```python
from build123d import *

# Parameters (mm, degrees)
SALIENTE_EXTRUIR1_DEPTH = 40
VACIADO1_T              = -1
SALIENTE_EXTRUIR3_START = 2
SALIENTE_EXTRUIR3_DEPTH = 2
CROQUIS5_R              = 3.75
CORTAR_EXTRUIR2_DEPTH   = 2.5
SALIENTE_EXTRUIR5_DEPTH = 5
CORTAR_EXTRUIR3_DEPTH   = 6
CORTAR_EXTRUIR4_DEPTH   = 1
CORTAR_EXTRUIR5_DEPTH   = 1


with BuildPart() as part:
    # Croquis1 → Saliente-Extruir1 (new body)
    with BuildSketch(Plane(origin=(0, 0, 0), x_dir=(1, 0, 0), z_dir=(0, 1, 0))):
        with BuildLine():
            Line((-25, 0), (-69.8, 0))
            ThreePointArc((-69.8, 0), (-64.717433049, 26.14754022), (-50.209918064, 48.487154258))
            Line((-50.209918064, 48.487154258), (-17.983495008, 17.366459261))
            ThreePointArc((-17.983495008, 17.366459261), (-23.179596364, 9.365164835), (-25, 0))
        make_face()
    extrude(amount=SALIENTE_EXTRUIR1_DEPTH)

    # Vaciado1
    vaciado1_openings = [part.faces().sort_by_distance(p)[0] for p in [
        (-46.068338787, 40, -18.61281705),
    ]]
    offset(amount=VACIADO1_T, openings=vaciado1_openings, kind=Kind.INTERSECTION)

    # Croquis4 → Saliente-Extruir3 (add)
    with BuildSketch(Plane.XZ.offset(SALIENTE_EXTRUIR3_START)):
        with BuildLine():
            Line((-25, 0), (-69.8, 0))
            ThreePointArc((-69.8, 0), (-64.717433049, -26.14754022), (-50.209918064, -48.487154258))
            Line((-50.209918064, -48.487154258), (-17.983495008, -17.366459261))
            ThreePointArc((-17.983495008, -17.366459261), (-23.179596364, -9.365164835), (-25, 0))
        make_face()
    extrude(amount=-SALIENTE_EXTRUIR3_DEPTH)

    # Croquis5 → Cortar-Extruir2 (cut)
    with BuildSketch(Plane(origin=(0, 1, 0), x_dir=(1, 0, 0), z_dir=(0, 1, 0))):
        with Locations(Location((-55.631031274, 22.476395605, 0), (0, 0, 270))):
            Circle(CROQUIS5_R)
    extrude(amount=-CORTAR_EXTRUIR2_DEPTH, mode=Mode.SUBTRACT)

    # Croquis6 → Saliente-Extruir5 (add)
    with BuildSketch(Plane(origin=(0, 1, 0), x_dir=(1, 0, 0), z_dir=(0, 1, 0))):
        with BuildLine():
            Line((-25, 0), (-50, 0))
            ThreePointArc((-50, 0), (-46.359192728, 18.730329671), (-35.966990017, 34.732918523))
            Line((-35.966990017, 34.732918523), (-17.983495008, 17.366459261))
            ThreePointArc((-17.983495008, 17.366459261), (-23.179596364, 9.365164835), (-25, 0))
        make_face()
    extrude(amount=SALIENTE_EXTRUIR5_DEPTH)

    # Croquis2 → Cortar-Extruir3 (cut)
    with BuildSketch(Plane(origin=(0, -2, 0), x_dir=(1, 0, 0), z_dir=(0, 1, 0))):
        with BuildLine():
            Line((-39.728874148, 27.818457163), (-29.899049617, 20.935539927))
            ThreePointArc((-29.899049617, 20.935539927), (-33.842210692, 13.67314066), (-36.050624432, 5.709857974))
            Line((-36.050624432, 5.709857974), (-47.902884519, 7.587071554))
            ThreePointArc((-47.902884519, 7.587071554), (-44.968416946, 18.168419781), (-39.728874148, 27.818457163))
        make_face()
    extrude(amount=CORTAR_EXTRUIR3_DEPTH, mode=Mode.SUBTRACT)

    # Croquis7 → Cortar-Extruir4 (cut)
    with BuildSketch(Plane.XY):
        Polygon((-62.8, 38), (-67.8, 35.113248654), (-67.8, 29.339745962), (-62.8, 26.452994616), (-57.8, 29.339745962), (-57.8, 35.113248654), align=None)
        Polygon((-47.8, 38), (-52.8, 35.113248654), (-52.8, 29.339745962), (-47.8, 26.452994616), (-42.8, 29.339745962), (-42.8, 35.113248654), align=None)
        Polygon((-32.8, 38), (-37.8, 35.113248654), (-37.8, 29.339745962), (-32.8, 26.452994616), (-27.8, 29.339745962), (-27.8, 35.113248654), align=None)
        Polygon((-47.8, 12.983724512), (-52.8, 10.096973166), (-52.8, 4.323470474), (-47.8, 1.436719129), (-42.8, 4.323470474), (-42.8, 10.096973166), align=None)
        Polygon((-32.8, 12.983724512), (-37.8, 10.096973166), (-37.8, 4.323470474), (-32.8, 1.436719129), (-27.8, 4.323470474), (-27.8, 10.096973166), align=None)
        Polygon((-62.8, 12.983724512), (-67.8, 10.096973166), (-67.8, 4.323470474), (-62.8, 1.436719129), (-57.8, 4.323470474), (-57.8, 10.096973166), align=None)
        Polygon((-55.299341949, 25.491862219), (-60.299670942, 22.605680781), (-60.300328993, 16.832178126), (-55.300658051, 13.94485691), (-50.300329058, 16.831038348), (-50.299671007, 22.604541002), align=None)
        Polygon((-40.177782617, 25.490568521), (-45.237770901, 22.710307401), (-45.359988284, 16.938098444), (-40.422217383, 13.946150607), (-35.362229099, 16.726411727), (-35.240011716, 22.498620684), align=None)
    extrude(amount=-CORTAR_EXTRUIR4_DEPTH, mode=Mode.SUBTRACT)

    # Croquis8 → Cortar-Extruir5 (cut)
    with BuildSketch(Plane(origin=(0, 0, 0), x_dir=(0.7193398003386502, 0, 0.6946583704589984), z_dir=(-0.6946583704589984, 0, 0.7193398003386502))):
        Polygon((-62.8, 38), (-67.8, 35.113248654), (-67.8, 29.339745962), (-62.8, 26.452994616), (-57.8, 29.339745962), (-57.8, 35.113248654), align=None)
        Polygon((-47.8, 38), (-52.8, 35.113248654), (-52.8, 29.339745962), (-47.8, 26.452994616), (-42.8, 29.339745962), (-42.8, 35.113248654), align=None)
        Polygon((-32.8, 38), (-37.8, 35.113248654), (-37.8, 29.339745962), (-32.8, 26.452994616), (-27.8, 29.339745962), (-27.8, 35.113248654), align=None)
        Polygon((-47.8, 12.983724512), (-52.8, 10.096973166), (-52.8, 4.323470474), (-47.8, 1.436719129), (-42.8, 4.323470474), (-42.8, 10.096973166), align=None)
        Polygon((-32.8, 12.983724512), (-37.8, 10.096973166), (-37.8, 4.323470474), (-32.8, 1.436719129), (-27.8, 4.323470474), (-27.8, 10.096973166), align=None)
        Polygon((-62.8, 12.983724512), (-67.8, 10.096973166), (-67.8, 4.323470474), (-62.8, 1.436719129), (-57.8, 4.323470474), (-57.8, 10.096973166), align=None)
        Polygon((-55.299341949, 25.491862219), (-60.299670942, 22.605680781), (-60.300328993, 16.832178126), (-55.300658051, 13.94485691), (-50.300329058, 16.831038348), (-50.299671007, 22.604541002), align=None)
        Polygon((-40.177782617, 25.490568521), (-45.237770901, 22.710307401), (-45.359988284, 16.938098444), (-40.422217383, 13.946150607), (-35.362229099, 16.726411727), (-35.240011716, 22.498620684), align=None)
    extrude(amount=CORTAR_EXTRUIR5_DEPTH, mode=Mode.SUBTRACT)


solid = part.part
```
Read the model definition and answer for the solid it produces. Units are mm, in the model's axes. Give positions to 0.01 mm unless a question says otherwise; leave off trailing zeros. Write each loop counter-clockwise with the first axis right and the second up, starting at its lowest first coordinate (ties: lowest second). Pieces come first, ordered by that corner, then holes. Notation, with made-up numbers: (86, 40) -> (91, 40) arc R20 ccw to (91, 55) -> close; hole circle Ø5 at (-5, -26.5). An arc over 180 degrees is marked (long way). Answer in a Markdown table with one row per item.
1) Section A-A on y = 9 is taken. Count the separate pieces of the cut face and the enclosed holes in it, plus the area to 3 significant figures.
Results list:
| item | result |
|---|---|
| separate pieces | 6 |
| enclosed holes | 0 |
| area | 98.4 mm^2 |
2) Determine the mould class of faces 1 (the flat face through (-39, 4, -17)), 2 (the flat face through (-43.744, 27.876, -41.558)), 3 (the cylindrical face through (-33.8, 0.96, -13.78)) for opening direction Y: released by +Y, released by -Y, zero draft, split by the parting line, or undercut.
Results list:
| item | result |
|---|---|
| face 1 | released by -Y |
| face 2 | undercut |
| face 3 | zero draft |
3) Straight lines are drawn through the part: line 1 (X direction, y = 2, z = -9.5); line 2 (X direction, y = 3.5, z = -19); line 3 (Z direction, x = -38, y = 11.5). For each, find the intervals that lie inside material, in ascending order. Write a range as [from, to].
Results list:
| item | result |
|---|---|
| line 1 | [-69.15, -68.14], [-49.09, -47.56], [-35.24, -23.12] |
| line 2 | [-67.16, -66.12], [-46.25, -44.62], [-31.16, -19.68] |
| line 3 | [-36.7, -35.31], [-1, 0] |
4) Each of these flat-tipped pins is pushed along its axis until it touches: pin 1 Ø1 at (y, z) = (9.5, -20.5) entering from +X; pin 2 Ø12 at (y, z) = (6.5, -8) entering from -X; pin 3 Ø8 at (x, z) = (-55, -23) entering from +Y. Where does it stop, or does it pass through?
Results list:
| item | result |
|---|---|
| pin 1 | x = -65.52 |
| pin 2 | x = -69.77 |
| pin 3 | y = 1 |
5) Section B-B on z = -20 is taken. Give the vertices of the cut face in (x, y).
Results list:
| item | result |
|---|---|
| outline | (-66.87, -2) -> (-44.18, -2) -> (-44.18, 4) -> (-30.53, 4) -> (-30.53, -2) -> (-20.71, -2) -> (-20.71, 3.75) -> (-22.15, 3.15) -> (-22.15, 6) -> (-45.83, 6) -> (-45.83, 1) -> (-52.82, 1) -> (-52.82, -1.5) -> (-58.45, -1.5) -> (-58.45, 1) -> (-65.83, 1) -> (-65.83, 40) -> (-66.87, 40) -> close; (-22.15, 11.27) -> (-20.71, 10.67) -> (-20.71, 28.77) -> (-22.15, 28.17) -> close; (-22.15, 36.28) -> (-20.71, 35.69) -> (-20.71, 40) -> (-22.15, 40) -> close |
6) Section D-D on y = 15 is taken. Give the vertices of the cut face in (x, z), plus the area to 3 significant figures.
Results list:
| item | result |
|---|---|
| outline | (-69.8, 0) arc R69.8 ccw to (-50.21, -48.49) -> (-41.09, -39.68) -> (-41.79, -38.96) -> (-50.18, -47.07) arc R68.8 cw to (-68.79, -1) -> (-57.13, -1) -> (-57.13, 0) -> close; (-53.47, -1) -> (-42.16, -1) -> (-42.16, 0) -> (-53.47, 0) -> close; (-39.16, -36.43) -> (-38.46, -37.15) -> (-30.33, -29.29) -> (-31.02, -28.57) -> close; (-38.5, -1) -> (-25.98, -1) arc R26 ccw to (-19.38, -17.33) -> (-28.39, -26.03) -> (-27.7, -26.75) -> (-17.98, -17.37) arc R25 cw to (-25, 0) -> (-38.5, 0) -> close |
| area | 144 mm^2 |
7) Section C-C on x = -58.5 is taken. Give the vertices of the cut face in (y, z).
Results list:
| item | result |
|---|---|
| outline | (-2, -38.08) -> (40, -38.08) -> (40, -36.21) -> (1, -36.21) -> (1, -24.89) -> (-1.5, -24.89) -> (-1.5, -20.06) -> (1, -20.06) -> (1, -1) -> (3.92, -1) -> (3.92, 0) -> (-2, 0) -> close; (10.5, -1) -> (15.79, -1) -> (15.79, 0) -> (10.5, 0) -> close; (23.64, -1) -> (28.94, -1) -> (28.94, 0) -> (23.64, 0) -> close; (35.52, -1) -> (40, -1) -> (40, 0) -> (35.52, 0) -> close |
